Verification items for this drawing (mm, ordinates from the low corner). A direction names the side the tool comes from. Round coordinates to 2 decimals unless told otherwise and drop trailing zeros. Order: outer loops, then holes, each group sorted by start corner. A loop starts at its lowest first (then second) coordinate and runs counter-clockwise, first axis right, second up. Notation, with made-up numbers: (45.5, 10.5) - (74.5, 10.5) arc R18 cw to (74.5, 39.5) - close; hole circle Ø11 at (67.5, 33.5). An arc over 180 degrees is marked (long way). Return JSON: item names as keys, results as strings. Group by question number.
Q1. Tool access check on the marked faces 1, 2 and 3. Record the directions out of +Z, -Z, +X, -X, +Y, -Y that give a thin tool (end or side, any length) a straight path to the whole face; none if there is none.
Q2. Sectioned sample at D-D, the plane y = 1.25. Record the cut outline in (x, z).
Q3. Gauge pin test, flat ends, axial feed: pin 1 Ø1 at (y, z) = (1.5, 1) entering from +X; pin 2 Ø5 at (x, y) = (20.5, 2) entering from -Z; pin 3 Ø1.5 at (x, y) = (27.5, 11) entering from -Z; pin 4 Ø1 at (y, z) = (1.5, 0.5) entering from -X. Record the tip position at first contact, or that the pin passes through.
Q4. Sectioned sample at B-B, the plane y = 11. Record the cut outline in (x, z) (3 decimals), then the cut area to 3 significant figures.
Q5. Sectioned sample at A-A, the plane z = 0.4. Record the cut outline in (x, y) (3 decimals).
Q6. Sectioned sample at C-C, the plane x = 24. Record the cut outline in (y, z), then the cut area to 3 significant figures.
Q7. Material ranges on line 1 along Y through (x, z) = (27.5, 1.65) (3 decimals); line 2 along X through (y, z) = (10, 1.2); line 3 along X through (y, z) = (11.5, 1), recorded low to high.
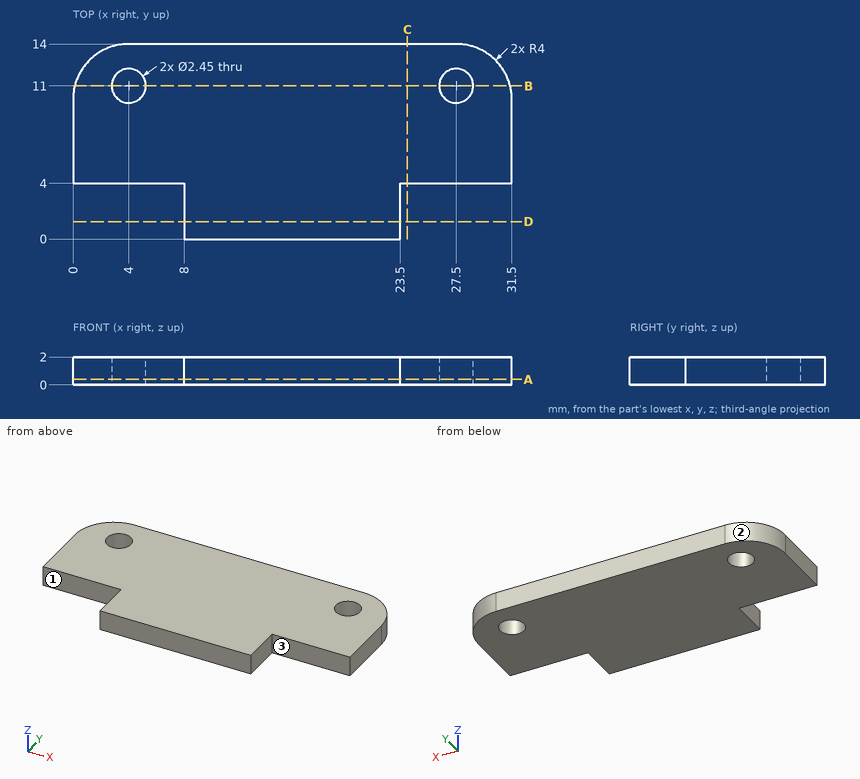
Reply:
{
 "1": {"face 1": "+Z, -Z, -X, -Y", "face 2": "+Z, -Z, -X, +Y", "face 3": "+Z, -Z, +X, -Y"},
 "2": {"outline": "(8, 0) - (23.5, 0) - (23.5, 2) - (8, 2) - close"},
 "3": {"pin 1": "x = 23.5", "pin 2": "z = 0", "pin 3": "through", "pin 4": "x = 8"},
 "4": {"outline": "(0.127, 0) - (2.775, 0) - (2.775, 2) - (0.127, 2) - close; (5.225, 0) - (26.275, 0) - (26.275, 2) - (5.225, 2) - close; (28.725, 0) - (31.373, 0) - (31.373, 2) - (28.725, 2) - close", "area": "52.7 mm^2"},
 "5": {"outline": "(0, 4) - (8, 4) - (8, 0) - (23.5, 0) - (23.5, 4) - (31.5, 4) - (31.5, 10) arc R4 ccw to (27.5, 14) - (4, 14) arc R4 ccw to (0, 10) - close; hole circle Ø2.45 at (4, 11); hole circle Ø2.45 at (27.5, 11)"},
 "6": {"outline": "(4, 0) - (14, 0) - (14, 2) - (4, 2) - close", "area": "20.0 mm^2"},
 "7": {"line 1": "4 to 9.775, 12.225 to 14", "line 2": "0 to 3.29, 4.71 to 26.79, 28.21 to 31.5", "line 3": "0.29 to 2.88, 5.12 to 26.38, 28.62 to 31.21"}
}
